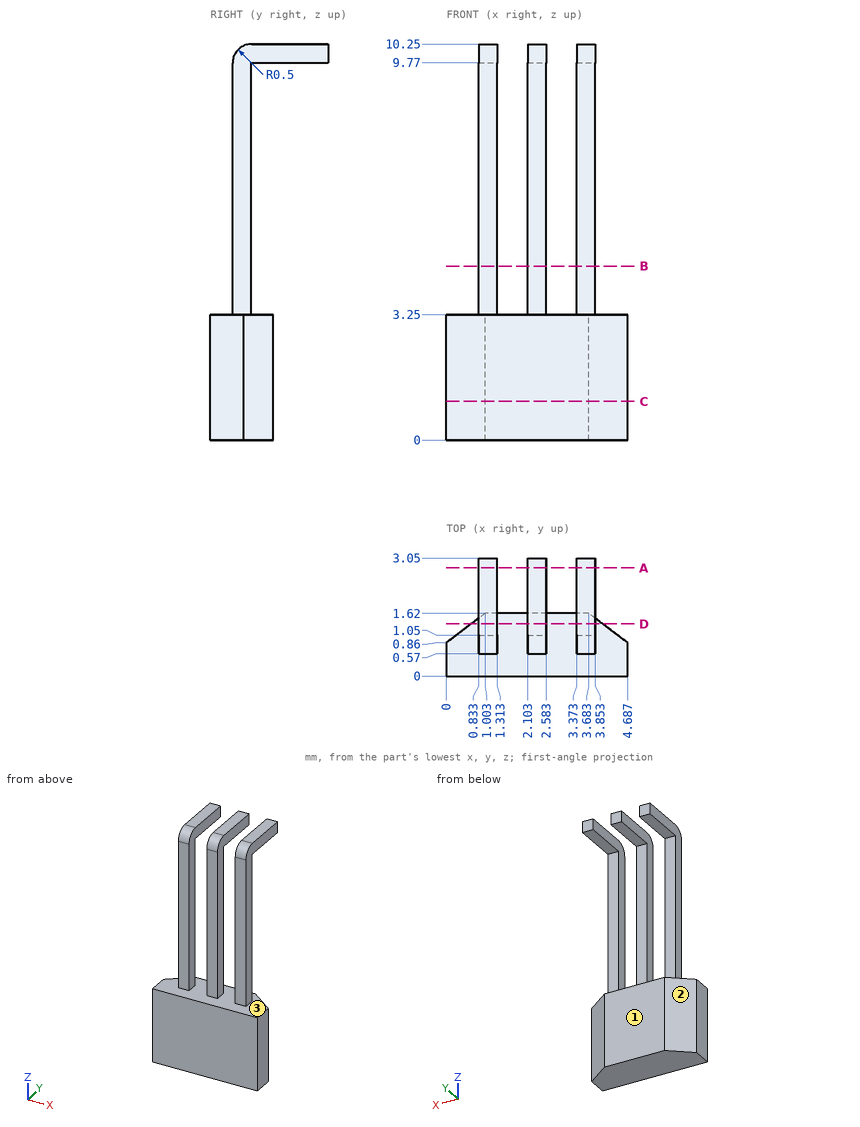
Verification items for this drawing (mm, ordinates from the low corner). Round coordinates to 2 decimals unless told otherwise and drop trailing zeros. Loops run counter-clockwise (first coordinate to the right, second up) from the corner with the lowest first, then second, coordinate; pieces in that order, holes last. Notation, with made-up numbers: (77.5, 20.5) - (99.5, 20.5) arc R19 cw to (99.5, 54.5) - close; hole circle Ø11 at (83.25, -27). An arc over 180 degrees is marked (long way). Answer as CSV lines item,"result". Start each with the question number.
Item 1: Depth check by flat-ended pin: P1, Ø0.5, axis at x = 2.5, z = 5.5, coming from the +Y side; P2, Ø1.2, axis at y = 1, z = 7.5, coming from the +X side; P3, Ø1.5, axis at y = 2.5, z = 6, coming from the +X side; P4, Ø1, axis at x = 3, z = 1.5, coming from the +Y side. Enter the tip coordinate at first touch or a pass-through.
Item 2: Section check D-D (y = 1.35). Record the boundary of the cut face in (x, z).
Item 3: Section check C-C (z = 1). Record the boundary of the cut face in (x, y).
Item 4: Scan lines: line 1 (X direction, y = 0.95, z = 6.5); line 2 (Z direction, x = 1.2, y = 2.5); line 3 (Z direction, x = 1, y = 0.3). Record each from-to range of solid material in increasing order. Write a range as [from, to].
Item 5: Section check A-A (y = 2.8). Record the boundary of the cut face in (x, z).
Item 6: Section check B-B (z = 4.5). Record the boundary of the cut face in (x, y).
Item 7: Release check for a two-part mould opening along X. For the marked faces 1, 2 and 3 record: +X half, -X half, draft (parallel to the pull), parting line (faces both ways), or undercut.
Report:
1,P1,"stops at y = 1.05"
1,P2,"stops at x = 3.85"
1,P3,"passes through"
1,P4,"stops at y = 1.62"
2,outline,"(0.65, 0) - (4.04, 0) - (4.04, 3.25) - (0.65, 3.25) - close; (0.83, 9.77) - (1.31, 9.77) - (1.31, 10.25) - (0.83, 10.25) - close; (2.1, 9.77) - (2.58, 9.77) - (2.58, 10.25) - (2.1, 10.25) - close; (3.37, 9.77) - (3.85, 9.77) - (3.85, 10.25) - (3.37, 10.25) - close"
3,outline,"(0, 0) - (4.69, 0) - (4.69, 0.86) - (3.68, 1.62) - (1, 1.62) - (0, 0.86) - close"
4,line 1,"x = [0.83, 1.31], [2.1, 2.58], [3.37, 3.85]"
4,line 2,"z = [9.77, 10.25]"
4,line 3,"z = [0, 3.25]"
5,outline,"(0.83, 9.77) - (1.31, 9.77) - (1.31, 10.25) - (0.83, 10.25) - close; (2.1, 9.77) - (2.58, 9.77) - (2.58, 10.25) - (2.1, 10.25) - close; (3.37, 9.77) - (3.85, 9.77) - (3.85, 10.25) - (3.37, 10.25) - close"
6,outline,"(0.83, 0.57) - (1.31, 0.57) - (1.31, 1.05) - (0.83, 1.05) - close; (2.1, 0.57) - (2.58, 0.57) - (2.58, 1.05) - (2.1, 1.05) - close; (3.37, 0.57) - (3.85, 0.57) - (3.85, 1.05) - (3.37, 1.05) - close"
7,face 1,"draft"
7,face 2,"-X half"
7,face 3,"undercut"
